```python
from build123d import *

# Parameters (mm, degrees)
F0_W     = 152.4
F0_H     = 76.2
F1_DEPTH = 19.05
F2_R     = 6.35
F3_DEPTH = 19.051
F4_W     = 19.05
F4_H     = 50.8
F6_SIZE  = 5.08
F7_W     = 10.795
F7_H     = 25.4
F9_SIZE2 = 5.07999
F9_SIZE  = 12.69999


# Not quite as in the source:
# - a fillet or chamfer is up to 0.001 mm smaller than in the source, because OpenCascade refuses the exact size


with BuildPart() as f1:
    # F0 (on Top) → F1 (new body)
    with BuildSketch(Plane.XY):
        Rectangle(F0_W, F0_H)
    extrude(amount=F1_DEPTH)

    # F2 (on Top) → F3 (cut, through all)
    with BuildSketch(Plane.XY):
        with Locations((-63.5, 25.4)):
            Circle(F2_R)
        with Locations((63.5, -25.4)):
            Circle(F2_R)
        with Locations((63.5, 25.4)):
            Circle(F2_R)
        with Locations((-63.5, -25.4)):
            Circle(F2_R)
    extrude(amount=F3_DEPTH, mode=Mode.SUBTRACT)

    # F4 (on Front) → F5 (revolve)
    with BuildSketch(Plane.XZ):
        with Locations((9.525, 44.45)):
            Rectangle(F4_W, F4_H)
    revolve(axis=Axis((0, 0, 44.45), (0, 0, -1)))

    # F6
    f6_edges = [f1.edges().sort_by_distance(p)[0] for p in [
        (0, -38.1, 19.05),
        (-76.2, 0, 19.05),
        (0, 38.1, 19.05),
        (76.2, 0, 19.05),
    ]]
    chamfer(f6_edges, length=F6_SIZE)

    # F7 (on Front) → F8 (revolve, cut)
    with BuildSketch(Plane.XZ):
        with Locations((13.6525, 44.45)):
            Rectangle(F7_W, F7_H)
    revolve(axis=Axis((0, 0, 19.05), (0, 0, 1)), mode=Mode.SUBTRACT)

    # F9 (size 12.7 and 5.08 in the source; OpenCascade refuses exactly that, so slightly less here)
    f9_edges = [f1.edges().sort_by_distance(p)[0] for p in [
        (-19.05, 0, 69.85),
    ]]
    f9_side = f1.faces().sort_by_distance((-19.05, 0, 63.5))[0]
    chamfer(f9_edges, length=F9_SIZE, length2=F9_SIZE2, reference=f9_side)


solid = f1.part
```
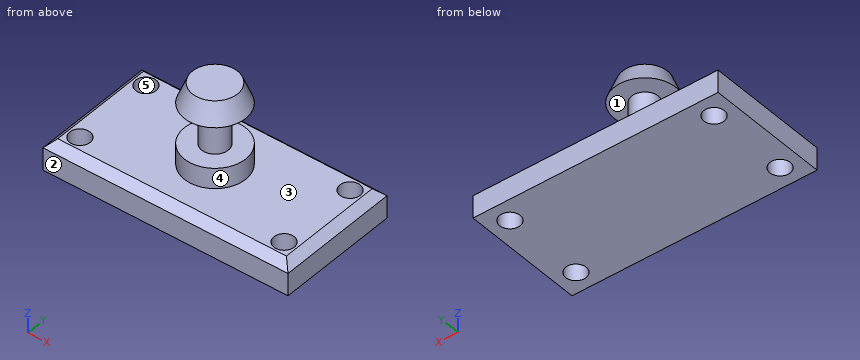
Source: CAD feature listing. Evaluate the final solid. Frame: model axes, mm. Face numbers are marked on the shaded views. A direction names the side the tool comes from. Round coordinates to 2 decimals unless told otherwise and drop trailing zeros. Loops run counter-clockwise (first coordinate to the right, second up) from the corner with the lowest first, then second, coordinate; pieces in that order, holes last. Notation, with made-up numbers: M -30,12.5 L -21,12.5 A22 ccw -21,30.5 Z; hole C -21,26 d11. An arc over 180 degrees is marked long. Use a Markdown table: item, result. Add a question column.
1. Cut plane D-D, the plane z = 25.5. Output: boundary loops of the cut face in (x, y), and give its area (3 significant figures).
2. Set-up query: the marked faces 1 and 2. Return all of +Z, -Z, +X, -X, +Y, -Y with unobstructed straight access to the full face (end or side cutting, diameter ignored); none if empty.
3. Ray query, line 1 along X through (y, z) = (25.4, 11.5); line 2 along Y through (x, z) = (-63, 8); line 3 along Y through (x, z) = (-63.5, 14.5). Return the intervals inside material, ascending. Write a range as [from, to].
4. Pull-direction query (X, two-part tool) for the marked faces 3, 4 and 5; classes: +X half, -X half, draft (parallel to the pull), parting line (faces both ways), or undercut.
5. Cut plane B-B, the plane y = -25.4. Output: boundary loops of the cut face in (x, z).
6. Cut plane A-A, the plane x = -63.5. Output: boundary loops of the cut face in (y, z).
7. Contact query for flat-ended pins moving along their axis: pin 1 (14.5 mm diameter, centred on x = 63.5, y = 25.4, fed in from -Z); pin 2 (12 mm diameter, centred on x = -52, y = -14.5, fed in from +Z). Output: stop coordinate, or through.
Solution:
| question | item | result |
|---|---|---|
| 1 | outline | C 0,0 d38.1 |
| 1 | area | 1,140 mm2 |
| 2 | face 1 | none |
| 2 | face 2 | +Z, -Z, +X, -X, -Y |
| 3 | line 1 | x = [-76.2, -69.85], [-57.15, 57.15], [69.85, 76.2] |
| 3 | line 2 | y = [-38.1, -31.73], [-19.07, 19.07], [31.73, 38.1] |
| 3 | line 3 | y = [-37.57, -31.75], [-19.05, 19.05], [31.75, 37.57] |
| 4 | face 3 | draft |
| 4 | face 4 | parting line |
| 4 | face 5 | undercut |
| 5 | outline | M -76.2,0 L -69.85,0 L -69.85,19.05 L -71.12,19.05 L -76.2,13.97 Z; M -57.15,0 L 57.15,0 L 57.15,19.05 L -57.15,19.05 Z; M 69.85,0 L 76.2,0 L 76.2,13.97 L 71.12,19.05 L 69.85,19.05 Z |
| 6 | outline | M -38.1,0 L -31.75,0 L -31.75,19.05 L -33.02,19.05 L -38.1,13.97 Z; M -19.05,0 L 19.05,0 L 19.05,19.05 L -19.05,19.05 Z; M 31.75,0 L 38.1,0 L 38.1,13.97 L 33.02,19.05 L 31.75,19.05 Z |
| 7 | pin 1 | stops at z = 0 |
| 7 | pin 2 | stops at z = 19.05 |
